Autodesk Inventor part; units mm, degrees
ref_plane "YZ Plane" through (0, 0, 0) normal (1, 0, 0) x (0, 1, 0)
ref_plane "XZ Plane" through (0, 0, 0) normal (0, 1, 0) x (-1, 0, 0)
ref_plane "XY Plane" through (0, 0, 0) normal (0, 0, 1) x (1, 0, 0)
sketch "Sketch1" plane through (0, 0, 0) normal (0, 1, 0) x (-1, 0, 0)
  line L0 (7.366, 6.1452) -> (7.366, -23.8548)
  line L1 (7.366, -23.8548) -> (0, -23.8548)
  line L2 (6.096, -8.0476) -> (6.096, -9.0212)
  line L3 (0, 0.4868) -> (0, 3.5348)
  line L4 (6.096, 3.5348) -> (6.096, -8.0476)
  line L5 (0, -9.0212) -> (0, -11.8152)
  line L6 (6.096, -12.0692) -> (6.096, -9.0212)
  line L7 (6.096, 3.5348) -> (0, 0.4868)
  line L8 (6.096, -12.0692) -> (0, -9.0212)
  line L9 (0, -23.8548) -> (0, -9.0212)
  line L10 (0, 0.4868) -> (0, 16.3788)
  line L11 (6.096, 13.3308) -> (6.096, 16.3788)
  line L12 (6.096, 13.3308) -> (0, 16.3788)
  line L13 (6.096, 28.9348) -> (6.096, 17.3524)
  line L14 (6.096, 28.9348) -> (0, 25.8868)
  line L15 (6.096, 17.3524) -> (6.096, 16.3788)
  line L16 (6.096, 38.7308) -> (6.096, 41.7788)
  line L17 (6.096, 38.7308) -> (0, 41.7788)
  line L18 (6.096, 54.3348) -> (6.096, 42.7524)
  line L19 (6.096, 54.3348) -> (0, 51.2868)
  line L20 (6.096, 42.7524) -> (6.096, 41.7788)
  line L21 (6.096, 64.1308) -> (6.096, 67.1788)
  line L22 (6.096, 64.1308) -> (0, 67.1788)
  line L23 (6.096, 79.7348) -> (6.096, 68.1524)
  line L24 (6.096, 79.7348) -> (0, 76.6868)
  line L25 (6.096, 68.1524) -> (6.096, 67.1788)
  line L26 (7.366, 6.1452) -> (7.366, 91.622)
  line L27 (7.366, 91.622) -> (0, 91.622)
  line L28 (0, 25.8868) -> (0, 41.7788)
  line L29 (0, 51.2868) -> (0, 67.1788)
  line L30 (0, 76.6868) -> (0, 91.622)
  line L31 (6.096, -4.2672) -> (4.0009, -4.2672) construction
  point P0 (0, 0)
  dimension "d0" = 7.366
  dimension "d8" = 9.508
  dimension "d10" = 3.048
  dimension "d11" = 3.048
  dimension "d12" = 6.096
  dimension "d17" = 25.4
  dimension "d24" = 11.7856
  dimension "d67" = 115.4768
  dimension "d70" = 23.8548
  dimension "d71" = 4.754
extrude "MultipleTeeth" add sketch "Sketch1" along normal blind 19.05
sketch "Sketch2" plane through (0, 0, 0) normal (0, -1, 0) x (1, 0, 0)
  line L0 (0, 0.4868) -> (-6.096, 3.5348) construction
  line L1 (-6.096, 3.5348) -> (-6.096, -12.0692) construction
  line L2 (-6.096, -12.0692) -> (0, -9.0212) construction
  line L3 (0, 16.3788) -> (0, 0.4868)
  line L4 (0, 0.4868) -> (-6.096, 3.5348)
  line L5 (-6.096, -12.0692) -> (0, -9.0212)
  line L6 (-6.096, 3.5348) -> (-6.096, -12.0692)
  line L7 (-6.096, -12.0692) -> (-6.096, 3.5348)
  line L8 (0, -9.0212) -> (-6.096, -12.0692)
  line L9 (-7.366, -23.8548) -> (-7.366, 91.622)
  line L10 (-7.366, -59.508) -> (-7.366, -32.8548)
  line L11 (-7.366, -23.8548) -> (0, -23.8548)
  line L12 (-7.366, 91.622) -> (0, 91.622)
  line L13 (-7.366, -55.8503) -> (-7.366, -40.458) construction
  line L14 (0, -43.0234) -> (0, -59.508) construction
  line L15 (-6.096, -62.0648) -> (0, -62.0648) construction
  line L16 (0, -32.8548) -> (0, -37.6258)
  line L17 (0, -49.9828) -> (0, -62.0648)
  line L18 (0, -62.0648) -> (0, -59.508)
  line L19 (0, -32.8548) -> (-7.366, -32.8548) construction
  line L20 (0, -51.9048) -> (-7.366, -51.9048) construction
  line L21 (0, -42.3798) -> (-7.366, -42.3798) construction
  line L22 (-6.096, -12.0692) -> (-6.096, -62.0648) construction
  line L23 (0, -37.6258) -> (-6.096, -34.5778)
  line L24 (-6.096, -50.1818) -> (-6.096, -34.5778)
  line L25 (0, -47.1338) -> (-6.096, -50.1818)
  line L26 (0, -9.0212) -> (0, -23.8548)
  line L27 (0, -23.8548) -> (0, -32.8548)
  line L28 (-7.366, -32.8548) -> (-7.366, -23.8548)
  line L29 (0, -49.9828) -> (0, -47.1338)
  line L30 (0, -62.0648) -> (-7.366, -62.0648)
  line L31 (-7.366, -62.0648) -> (-7.366, -59.508)
  point P0 (0, 0)
  dimension "d25" = 115.4768
  dimension "d33" = 9
  dimension "d34" = 19.05
  dimension "d36" = 9.525
  dimension "d38" = 10.16
extrude "LongTooth" add sketch "Sketch2" against normal blind 100.2792
sketch "Sketch3" plane through (0, 19.05, 0) normal (0, 1, 0) x (1, 0, 0)
  line L0 (-6.096, -3.5348) -> (-6.096, 12.0692) construction
  line L1 (0, 23.8548) -> (-7.366, 23.8548)
  line L2 (-7.366, -91.622) -> (0, -91.622)
  line L3 (-7.366, 23.8548) -> (-6.096, 23.8548)
  line L4 (-6.096, 23.8548) -> (-6.096, -91.622)
  line L5 (-6.096, -91.622) -> (-7.366, -91.622)
  line L6 (-7.366, -91.622) -> (-7.366, 23.8548)
  point P0 (0, 0)
extrude "ThinPlate" add sketch "Sketch3" along normal up to surface (81.2292 mm away)
sketch "Sketch4" plane through (0, 0, 0) normal (0, -1, 0) x (1, 0, 0)
  line L0 (-6.096, 91.622) -> (0, 91.622)
  line L1 (-7.366, 91.622) -> (-7.366, -62.0648)
  line L2 (0, 91.622) -> (-7.366, 91.622)
  line L3 (-7.366, 91.622) -> (-7.366, -62.0648)
  line L4 (-7.366, -62.0648) -> (0, -62.0648)
  line L5 (0, -62.0648) -> (0, 91.622)
  point P0 (0, 0)
extrude "Extrusion4" add sketch "Sketch4" along normal blind 5.08
ref_plane "Work Plane1" through (-15.892, 0, 8.4328) normal (0, 0, 1) x (0, 1, 0)
sketch "Sketch6" plane through (0, 19.05, 16.3788) normal (1, 0, 0) x (0, 0, -1)
  circle A0 centre (71.4586, -8.89) radius 1.9304
  line L0 (78.4436, 81.2292) -> (78.4436, -24.13)
  line L1 (78.4436, -24.13) -> (-75.2432, -24.13)
  circle A1 centre (58.7586, -8.89) radius 1.9304
  circle A2 centre (46.0586, -8.89) radius 1.9304
  circle A3 centre (71.4586, 3.81) radius 1.9304
  circle A4 centre (58.7586, 3.81) radius 1.9304
  circle A5 centre (46.0586, 3.81) radius 1.9304
  circle A6 centre (71.4586, 16.51) radius 1.9304
  circle A7 centre (58.7586, 16.51) radius 1.9304
  circle A8 centre (46.0586, 16.51) radius 1.9304
  circle A9 centre (71.4586, 29.21) radius 1.9304
  circle A10 centre (58.7586, 29.21) radius 1.9304
  circle A11 centre (46.0586, 29.21) radius 1.9304
  circle A12 centre (71.4586, 41.91) radius 1.9304
  circle A13 centre (58.7586, 41.91) radius 1.9304
  circle A14 centre (46.0586, 41.91) radius 1.9304
  circle A15 centre (71.4586, 54.61) radius 1.9304
  circle A16 centre (58.7586, 54.61) radius 1.9304
  circle A17 centre (46.0586, 54.61) radius 1.9304
  circle A18 centre (71.4586, 67.31) radius 1.9304
  circle A19 centre (58.7586, 67.31) radius 1.9304
  circle A20 centre (46.0586, 67.31) radius 1.9304
  circle A21 centre (33.3586, -8.89) radius 1.9304
  circle A22 centre (33.3586, 3.81) radius 1.9304
  circle A23 centre (33.3586, 16.51) radius 1.9304
  circle A24 centre (33.3586, 29.21) radius 1.9304
  circle A25 centre (33.3586, 41.91) radius 1.9304
  circle A26 centre (33.3586, 54.61) radius 1.9304
  circle A27 centre (33.3586, 67.31) radius 1.9304
  circle A28 centre (20.6586, -8.89) radius 1.9304
  circle A29 centre (20.6586, 3.81) radius 1.9304
  circle A30 centre (20.6586, 16.51) radius 1.9304
  circle A31 centre (20.6586, 29.21) radius 1.9304
  circle A32 centre (20.6586, 41.91) radius 1.9304
  circle A33 centre (20.6586, 54.61) radius 1.9304
  circle A34 centre (20.6586, 67.31) radius 1.9304
  circle A35 centre (7.9586, -8.89) radius 1.9304
  circle A36 centre (7.9586, 3.81) radius 1.9304
  circle A37 centre (7.9586, 16.51) radius 1.9304
  circle A38 centre (7.9586, 29.21) radius 1.9304
  circle A39 centre (7.9586, 41.91) radius 1.9304
  circle A40 centre (7.9586, 54.61) radius 1.9304
  circle A41 centre (7.9586, 67.31) radius 1.9304
  circle A42 centre (-4.7414, -8.89) radius 1.9304
  circle A43 centre (-4.7414, 3.81) radius 1.9304
  circle A44 centre (-4.7414, 16.51) radius 1.9304
  circle A45 centre (-4.7414, 29.21) radius 1.9304
  circle A46 centre (-4.7414, 41.91) radius 1.9304
  circle A47 centre (-4.7414, 54.61) radius 1.9304
  circle A48 centre (-4.7414, 67.31) radius 1.9304
  circle A49 centre (-17.4414, -8.89) radius 1.9304
  circle A50 centre (-17.4414, 3.81) radius 1.9304
  circle A51 centre (-17.4414, 16.51) radius 1.9304
  circle A52 centre (-17.4414, 29.21) radius 1.9304
  circle A53 centre (-17.4414, 41.91) radius 1.9304
  circle A54 centre (-17.4414, 54.61) radius 1.9304
  circle A55 centre (-17.4414, 67.31) radius 1.9304
  circle A56 centre (-30.1414, -8.89) radius 1.9304
  circle A57 centre (-30.1414, 3.81) radius 1.9304
  circle A58 centre (-30.1414, 16.51) radius 1.9304
  circle A59 centre (-30.1414, 29.21) radius 1.9304
  circle A60 centre (-30.1414, 41.91) radius 1.9304
  circle A61 centre (-30.1414, 54.61) radius 1.9304
  circle A62 centre (-30.1414, 67.31) radius 1.9304
  circle A63 centre (-42.8414, -8.89) radius 1.9304
  circle A64 centre (-42.8414, 3.81) radius 1.9304
  circle A65 centre (-42.8414, 16.51) radius 1.9304
  circle A66 centre (-42.8414, 29.21) radius 1.9304
  circle A67 centre (-42.8414, 41.91) radius 1.9304
  circle A68 centre (-42.8414, 54.61) radius 1.9304
  circle A69 centre (-42.8414, 67.31) radius 1.9304
  circle A70 centre (-55.5414, -8.89) radius 1.9304
  circle A71 centre (-55.5414, 3.81) radius 1.9304
  circle A72 centre (-55.5414, 16.51) radius 1.9304
  circle A73 centre (-55.5414, 29.21) radius 1.9304
  circle A74 centre (-55.5414, 41.91) radius 1.9304
  circle A75 centre (-55.5414, 54.61) radius 1.9304
  circle A76 centre (-55.5414, 67.31) radius 1.9304
  circle A77 centre (-68.2414, -8.89) radius 1.9304
  circle A78 centre (-68.2414, 3.81) radius 1.9304
  circle A79 centre (-68.2414, 16.51) radius 1.9304
  circle A80 centre (-68.2414, 29.21) radius 1.9304
  circle A81 centre (-68.2414, 41.91) radius 1.9304
  circle A82 centre (-68.2414, 54.61) radius 1.9304
  circle A83 centre (-68.2414, 67.31) radius 1.9304
  point P0 (16.3788, -19.05)
  dimension "d56" = 3.8608
  dimension "d57" = 6.985
  dimension "d58" = 15.24
  dimension "d61" = 12.7
  dimension "d64" = 12.7
extrude "Extrusion5" cut sketch "Sketch6" against normal through all contours A0 | A2 | A6 | A8 | A12 | A14 | A18 | A20 | A21 | A23 | A25 | A27 | A35 | A37 | A39 | A41 | A49 | A51 | A53 | A55 | A63 | A65 | A67 | A69 | A77 | A79 | A81 | A83
sketch "Sketch7" plane through (0, 19.05, 16.3788) normal (1, 0, 0) x (0, 0, -1)
  circle A0 centre (-68.2414, -8.89) radius 1.9304
  circle A1 centre (-68.2414, -8.89) radius 4.445
  circle A2 centre (-42.8414, -8.89) radius 1.9304
  circle A3 centre (-42.8414, -8.89) radius 4.445
  circle A4 centre (-17.4414, -8.89) radius 1.9304
  circle A5 centre (-17.4414, -8.89) radius 4.445
  circle A6 centre (7.9586, -8.89) radius 1.9304
  circle A7 centre (7.9586, -8.89) radius 4.445
  circle A8 centre (33.3586, -8.89) radius 1.9304
  circle A9 centre (33.3586, -8.89) radius 4.445
  circle A10 centre (46.0586, -8.89) radius 1.9304
  circle A11 centre (46.0586, -8.89) radius 4.445
  circle A12 centre (71.4586, -8.89) radius 1.9304
  circle A13 centre (71.4586, -8.89) radius 4.445
  circle A14 centre (46.0586, 16.51) radius 1.9304
  circle A15 centre (46.0586, 16.51) radius 4.445
  circle A16 centre (71.4586, 16.51) radius 1.9304
  circle A17 centre (71.4586, 16.51) radius 4.445
  circle A18 centre (46.0586, 41.91) radius 1.9304
  circle A19 centre (46.0586, 41.91) radius 4.445
  circle A20 centre (71.4586, 41.91) radius 1.9304
  circle A21 centre (71.4586, 41.91) radius 4.445
  circle A22 centre (46.0586, 67.31) radius 1.9304
  circle A23 centre (46.0586, 67.31) radius 4.445
  circle A24 centre (71.4586, 67.31) radius 4.445
  point P0 (16.3788, -19.05)
  dimension "d74" = 8.89
  dimension "d75" = 8.89
  dimension "d76" = 8.89
  dimension "d77" = 8.89
  dimension "d78" = 8.89
  dimension "d79" = 8.89
  dimension "d80" = 8.89
  dimension "d81" = 8.89
  dimension "d82" = 8.89
  dimension "d83" = 8.89
  dimension "d84" = 8.89
  dimension "d85" = 8.89
  dimension "d86" = 8.89
extrude "Extrusion6" cut sketch "Sketch7" against normal blind 2.8194 contours A0 | A1 | A2 | A3 | A4 | A5 | A6 | A7 | A8 | A9 | A10 | A11 | A12 | A13 | A14 | A15 | A16 | A17 | A18 | A19 | A20 | A21 | A22 | A23 | A24
equation "\"d11\" = d10"
equation "\"d71\" = 0.5 * d8"
equation "\"d36\" = 0.5 * d34"
properties part number "Lift mount receiver left"
Could you check a few things on this model? Use its own coordinates, in mm. A direction names the side the tool comes from. Give positions to 0.01 mm unless a question says otherwise; leave off trailing zeros. Order: outer loops, then holes, each group sorted by start corner. A loop starts at its lowest first (then second) coordinate and runs counter-clockwise, first axis right, second up. Notation, with made-up numbers: (-38, 48.5) - (14, 48.5) arc R22 cw to (14, 75.5) - close; hole circle Ø11 at (80.5, -30.5). An arc over 180 degrees is marked (long way). Return JSON: item names as keys, results as strings. Group by question number.
Q1. Will these pins go through, and if not, where does the flat tip stop? pin 1 Ø4.5 at (y, z) = (10.16, 84.62) entering from -X; pin 2 Ø3 at (x, z) = (-4, 73) entering from +Y; pin 3 Ø5.5 at (y, z) = (86.36, -55.08) entering from +X; pin 4 Ø2.5 at (y, z) = (10.16, -55.08) entering from -X.
Q2. Thinking about a two-plate mould opening in X: for faces 4 (the face through (-3.091, 9.392, 40.233)), 5 (the face through (-6.7, 88, 7.4)), 6 (the face through (-2.819, 84, -31)), which applies, pulls with the +X half, pulls with the -X half, needs draft (parallel to the pull), parting line crosses it, or undercut?
Q3. Suppose I cut it at A-A, the plane y = 69. Please give me the cut outline in (x, z), and give its area (3 significant figures).
Q4. Suppose I cut it at B-B, the plane z = 23. Please give me the cut outline in (x, y), and give its area (3 significant figures).
Q5. Suppose I cut it at C-C, the plane y = 10.16. State how many separate pieces and enclosed holes the cut face has, and give its area (3 significant figures).
Q6. Which directions (+Z, -Z, +X, -X, +Y, -Y) give clear straight access to the entire face, cutting with the end or side of a thin tool? Please do faces 1 (the face through (-6.722, 87.665, 35.243)), 2 (the face through (-1.39, 39.31, -57.47)), 3 (the face through (-3, 19.05, -16)).
Q7. Please list where these lines run through material, in increasing order: line 1 along Z through (x, y) = (-1.75, 33); line 2 along X through (y, z) = (23, 79); line 3 along Y through (x, z) = (-5.75, 67). Write a range as [from, to].
Resolved:
{
 "1": {"pin 1": "stops at x = -7.37", "pin 2": "stops at y = 0", "pin 3": "stops at x = -2.82", "pin 4": "passes through"},
 "2": {"face 4": "undercut", "face 5": "needs draft", "face 6": "pulls with the +X half"},
 "3": {"outline": "(-7.37, -62.06) - (0, -62.06) - (0, -47.13) - (-6.1, -50.18) - (-6.1, -34.58) - (0, -37.63) - (0, -23.85) - (-6.1, -23.85) - (-6.1, 91.62) - (-7.37, 91.62) - close", "area": "352 mm2"},
 "4": {"outline": "(-7.37, -5.08) - (0, -5.08) - (0, 0) - (-6.1, 0) - (-6.1, 100.28) - (-7.37, 100.28) - close", "area": "165 mm2"},
 "5": {"separate pieces": "8", "enclosed holes": "0", "area": "451 mm2"},
 "6": {"face 1": "+X, -X", "face 2": "+X", "face 3": "+Z, +X, +Y"},
 "7": {"line 1": "z = [-62.06, -58.71], [-51.45, -48.01], [-36.75, -33.31], [-26.05, -23.85]", "line 2": "x = [-7.37, -6.1]", "line 3": "y = [-5.08, 0]"}
}
